```python
from build123d import *

# Parameters (mm, degrees)
CROQUIS1_R              = 22
SALIENTE_EXTRUIR1_DEPTH = 5
CROQUIS2_R              = 2.05
CROQUIS2_R_2            = 2.065143699
CROQUIS2_R_3            = 1.702015819
CORTAR_EXTRUIR1_DEPTH   = 5
CROQUIS3_W              = 34
CROQUIS3_H              = 25
SALIENTE_EXTRUIR2_DEPTH = 48
SALIENTE_EXTRUIR3_DEPTH = 25
CORTAR_EXTRUIR2_DEPTH   = 19.346
CROQUIS6_R              = 2.049356991
CROQUIS6_R_2            = 2.05
CROQUIS6_W              = 22
CROQUIS6_H              = 42
CORTAR_EXTRUIR3_DEPTH   = 19.346
CORTAR_EXTRUIR4_DEPTH   = 49.346


with BuildPart() as part:
    # Croquis1 → Saliente-Extruir1 (new body)
    with BuildSketch(Plane(origin=(0, 0, 0), x_dir=(1, 0, 0), z_dir=(0, 1, 0))):
        with Locations(Location((0, 0, 0), (0, 0, 270))):
            Circle(CROQUIS1_R)
    extrude(amount=SALIENTE_EXTRUIR1_DEPTH)

    # Croquis2 → Cortar-Extruir1 (cut)
    with BuildSketch(Plane(origin=(0, 5, 0), x_dir=(1, 0, 0), z_dir=(0, 1, 0))):
        with Locations(Location((0, 17.5, 0), (0, 0, 270))):
            Circle(CROQUIS2_R)
        with Locations(Location((-7, -15.999727998, 0), (0, 0, 270))):
            Circle(CROQUIS2_R_2)
        with Locations(Location((7, -15.999727998, 0), (0, 0, 270))):
            Circle(CROQUIS2_R_3)
    extrude(amount=-CORTAR_EXTRUIR1_DEPTH, mode=Mode.SUBTRACT)

    # Croquis3 → Saliente-Extruir2 (add)
    with BuildSketch(Plane(origin=(0, 5, 0), x_dir=(1, 0, 0), z_dir=(0, 1, 0))):
        Rectangle(CROQUIS3_W, CROQUIS3_H)
    extrude(amount=SALIENTE_EXTRUIR2_DEPTH)

    # Croquis4 → Saliente-Extruir3 (add)
    with BuildSketch(Plane(origin=(0, 0, -12.5), x_dir=(-1, 0, 0), z_dir=(0, 0, -1))):
        with BuildLine():
            Line((-17, 53), (17, 53))
            ThreePointArc((17, 53), (0, 70), (-17, 53))
        make_face()
    extrude(amount=-SALIENTE_EXTRUIR3_DEPTH)

    # Croquis5 → Cortar-Extruir2 (cut)
    with BuildSketch(Plane.XY.offset(12.5)):
        with BuildLine():
            Line((14.5, 7.5), (14.5, 53))
            ThreePointArc((14.5, 53), (0, 67.5), (-14.5, 53))
            Line((-14.5, 53), (-14.5, 7.5))
            Line((-14.5, 7.5), (14.5, 7.5))
        make_face()
    extrude(amount=-CORTAR_EXTRUIR2_DEPTH, mode=Mode.SUBTRACT)

    # Croquis6 → Cortar-Extruir3 (cut)
    with BuildSketch(Plane.XY.offset(-6.846)):
        with Locations((-5, 12.250643009)):
            Circle(CROQUIS6_R)
        with Locations((5, 12.250643009)):
            Circle(CROQUIS6_R)
        with Locations((-5, 61.75)):
            Circle(CROQUIS6_R_2)
        with Locations((5, 61.75)):
            Circle(CROQUIS6_R_2)
        with Locations((0, 37)):
            Rectangle(CROQUIS6_W, CROQUIS6_H)
    extrude(amount=-CORTAR_EXTRUIR3_DEPTH, mode=Mode.SUBTRACT)

    # Croquis7 → Cortar-Extruir4 (cut)
    with BuildSketch(Plane(origin=(17, 0, 0), x_dir=(0, 0, -1), z_dir=(1, 0, 0))):
        Polygon((-12.5, 53), (0.054068921, 53), (10.400499838, 92.559180941), (-12.5, 92.559180941), align=None)
        Polygon((-12.5, 53), (-12.5, 5), (0.054068921, 53), align=None)
    extrude(amount=-CORTAR_EXTRUIR4_DEPTH, mode=Mode.SUBTRACT)


solid = part.part
```
Geometry: final body of the model. Coordinates: model frame, mm. A direction names the side the tool comes from. Round coordinates to 2 decimals unless told otherwise and drop trailing zeros. Write each loop counter-clockwise with the first axis right and the second up, starting at its lowest first coordinate (ties: lowest second). Pieces come first, ordered by that corner, then holes.
Item 1: Section query B-B (z = -5.5). Return loops of the section in (x, y), plus the area to 3 significant figures.
Item 2: Material intervals for L1, parallel to Y at x = 5, z = -10; L2, parallel to X at y = 15, z = -5.5; L3, parallel to Z at x = -12, y = 61, sorted ascending.
Item 3: Section query D-D (y = 65). Return loops of the section in (x, z).
Item 4: Section query A-A (x = 1). Return loops of the section in (y, z), plus the area to 3 significant figures.
Item 5: Section query C-C (z = 5). Return loops of the section in (x, y).
Item 6: Mould query, pull axis X, two halves, no side actions, for faces 6 (the face through (0, 5, 14)), 7 (the face through (0.319, 67.496, -4.157)), 8 (the face through (-17, 29, -3)), 9 (the face through (-21.477, 2.465, -4.769)). Classes: +X half, -X half, draft (parallel to the pull), parting line (faces both ways), or undercut.
Item 7: Set-up query: faces 1 (the face through (14.5, 25, 1)), 2 (the face through (12, 38, -12.5)), 3 (the face through (-11, 37, -10)), 4 (the face through (0, 0, 0)), 5 (the face through (0, 70, -8)). Return all of +Z, -Z, +X, -X, +Y, -Y with unobstructed straight access to the full face (end or side cutting, diameter ignored); none if empty.
Item 8: Pin query (flat end, axial travel): P1, Ø20, axis at y = 19, z = 6, coming from the +X side; P2, Ø1.7, axis at x = 3, z = -9, coming from the +Y side; P3, Ø20, axis at y = 17.5, z = -3.5, coming from the -X side; P4, Ø1.5, axis at x = 8.5, z = -11, coming from the -Y side. Return the tip coordinate at first contact, or that it passes through.
Completed:
1. outline: (-21.3, 0) - (21.3, 0) - (21.3, 5) - (17, 5) - (17, 53) arc R17 ccw to (-17, 53) - (-17, 5) - (-21.3, 5) - close; hole (-14.5, 7.5) - (14.5, 7.5) - (14.5, 53) arc R14.5 ccw to (-14.5, 53) - close
1. area: 649 mm2
2. L1: y = 0 to 10.2, 14.3 to 16, 58 to 59.7, 63.8 to 69.25
2. L2: x = -17 to -14.5, 14.5 to 17
2. L3: z = -12.5 to -6.85
3. outline: (-12.04, -12.5) - (12.04, -12.5) - (12.04, -3.19) - (8.14, -3.19) - (8.14, -6.85) - (-8.14, -6.85) - (-8.14, -3.19) - (-12.04, -3.19) - close
4. outline: (0, -21.98) - (5, -21.98) - (5, -19.29) - (0, -19.29) - close; (0, -15.71) - (5, -15.71) - (5, -12.5) - (16, -12.5) - (16, -6.85) - (7.5, -6.85) - (7.5, 11.85) - (5, 12.5) - (5, 21.98) - (0, 21.98) - close; (58, -12.5) - (69.97, -12.5) - (69.97, -4.49) - (67.47, -3.84) - (67.47, -6.85) - (58, -6.85) - close
4. area: 386 mm2
5. outline: (-21.42, 0) - (21.42, 0) - (21.42, 5) - (17, 5) - (17, 33.68) - (14.5, 33.68) - (14.5, 7.5) - (-14.5, 7.5) - (-14.5, 33.68) - (-17, 33.68) - (-17, 5) - (-21.42, 5) - close
6. face 6: draft
6. face 7: undercut
6. face 8: -X half
6. face 9: parting line
7. face 1: +Z
7. face 2: -Z, +X, -X, +Y
7. face 3: +Z, -Z
7. face 4: +Z, -Z, +X, -X, -Y
7. face 5: +Z, -Z, +Y
8. P1: stops at x = 17
8. P2: stops at y = 69.86
8. P3: stops at x = -17
8. P4: stops at y = 0
